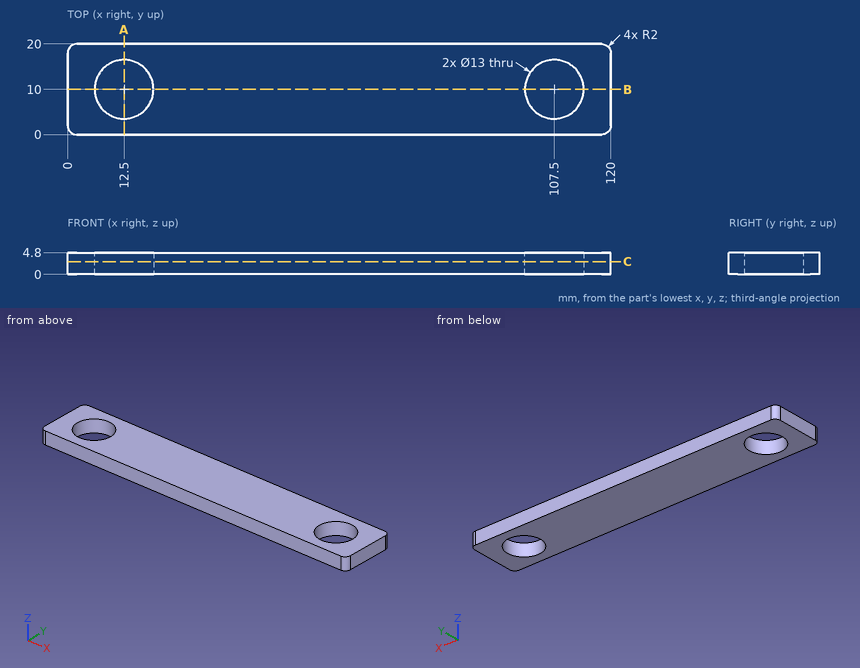
Design review of the part shown in the three views and the two pictorial views. Dimensions are in mm from the part's minimum x, y and z. Round coordinates to 2 decimals unless told otherwise and drop trailing zeros. Loops run counter-clockwise (first coordinate to the right, second up) from the corner with the lowest first, then second, coordinate; pieces in that order, holes last.
(1) We need section B-B (y = 10). Give the boundary of the cut face in (x, z), plus the area to 3 significant figures.
Returned:
outline: (0, 0) - (6, 0) - (6, 4.8) - (0, 4.8) - close; (19, 0) - (101, 0) - (101, 4.8) - (19, 4.8) - close; (114, 0) - (120, 0) - (120, 4.8) - (114, 4.8) - close
area: 451 mm2
(2) We need section C-C (z = 2.8). Give the boundary of the cut face in (x, y), plus the area to 3 significant figures.
Returned:
outline: (0, 2) arc R2 ccw to (2, 0) - (118, 0) arc R2 ccw to (120, 2) - (120, 18) arc R2 ccw to (118, 20) - (2, 20) arc R2 ccw to (0, 18) - close; hole circle Ø13 at (12.5, 10); hole circle Ø13 at (107.5, 10)
area: 2,130 mm2
(3) Wall thickness on line 1 along X through (y, z) = (8, 1.45); line 2 along X through (y, z) = (8.75, 2.45); line 3 along Y through (x, z) = (107.5, 1.8): over which ranges is each line inside the solid? List them lowest first.
Returned:
line 1: x = 0 to 6.32, 18.68 to 101.32, 113.68 to 120
line 2: x = 0 to 6.12, 18.88 to 101.12, 113.88 to 120
line 3: y = 0 to 3.5, 16.5 to 20
(4) We need section A-A (x = 12.5). Give the boundary of the cut face in (y, z).
Returned:
outline: (0, 0) - (3.5, 0) - (3.5, 4.8) - (0, 4.8) - close; (16.5, 0) - (20, 0) - (20, 4.8) - (16.5, 4.8) - close
